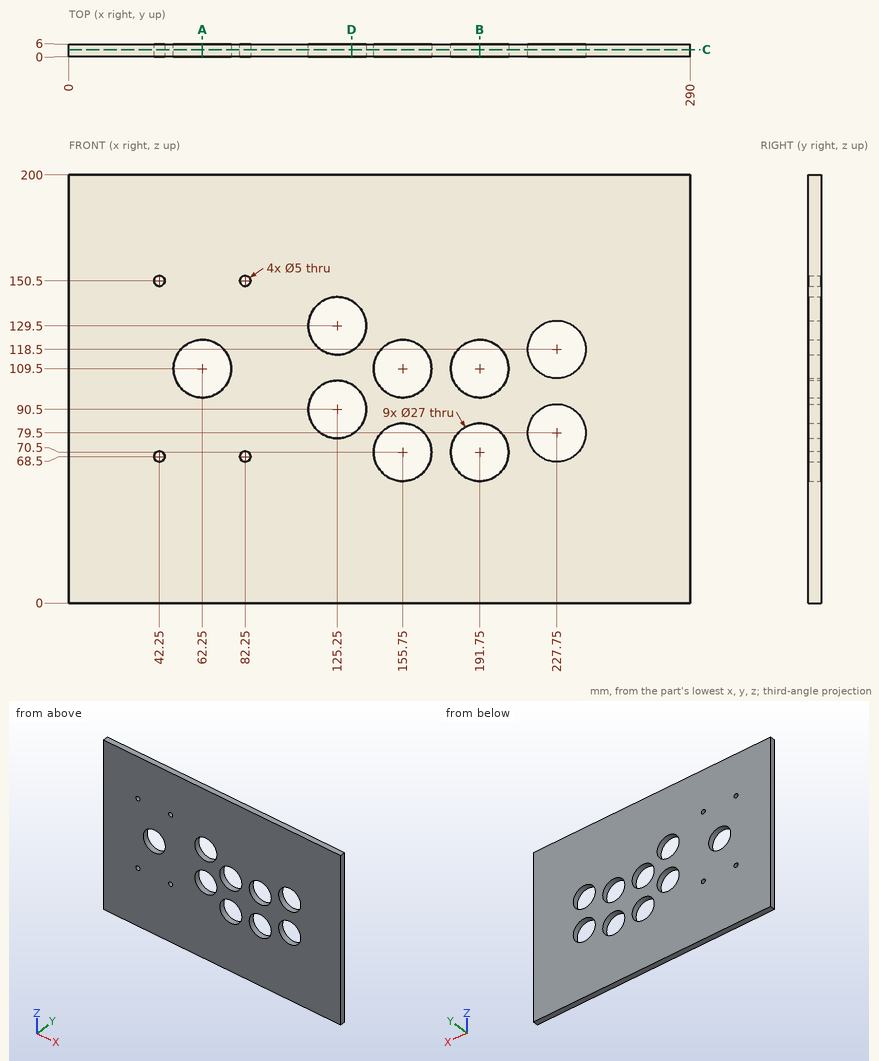
Input: dimensioned drawing with shaded views. Units: mm. Origin: part minimum x, y, z. Coordinates: 2 decimals unless noted, no trailing zeros. Loops run counter-clockwise (first coordinate to the right, second up) from the corner with the lowest first, then second, coordinate; pieces in that order, holes last. Notation, with made-up numbers: M -33.75,-39 L 25.25,-39 A27 cw 25.25,-4 Z; hole C 47,38.25 d8. An arc over 180 degrees is marked long. Put each result on its own line as item: value.
(1) Cut plane A-A on x = 62.25. Return the cut outline in (y, z), then the cut area to 3 significant figures.
Answer sheet:
outline: M 0,0 L 6,0 L 6,96 L 0,96 Z; M 0,123 L 6,123 L 6,200 L 0,200 Z
area: 1,040 mm^2
(2) Cut plane B-B on x = 191.75. Return the cut outline in (y, z).
Answer sheet:
outline: M 0,0 L 6,0 L 6,57 L 0,57 Z; M 0,84 L 6,84 L 6,96 L 0,96 Z; M 0,123 L 6,123 L 6,200 L 0,200 Z
(3) Cut plane C-C on y = 3.4. State how many separate pieces and enclosed holes the cut face has, then the cut area to 3 significant figures.
Answer sheet:
separate pieces: 1
enclosed holes: 13
area: 52,800 mm^2
(4) Cut plane D-D on x = 132. Return the cut outline in (y, z), then the cut area to 3 significant figures.
Answer sheet:
outline: M 0,0 L 6,0 L 6,78.81 L 0,78.81 Z; M 0,102.19 L 6,102.19 L 6,117.81 L 0,117.81 Z; M 0,141.19 L 6,141.19 L 6,200 L 0,200 Z
area: 919 mm^2
(5) Material intervals for probe 1 along Z at (x, y) = (191.75, 3.4); probe 2 along Z at (x, y) = (125.25, 1.3); probe 3 along X at (y, z) = (2.05, 109), sorted ascending.
Answer sheet:
probe 1: z = 0 to 57, 84 to 96, 123 to 200
probe 2: z = 0 to 77, 104 to 116, 143 to 200
probe 3: x = 0 to 48.76, 75.74 to 142.26, 169.24 to 178.26, 205.24 to 218.16, 237.34 to 290
